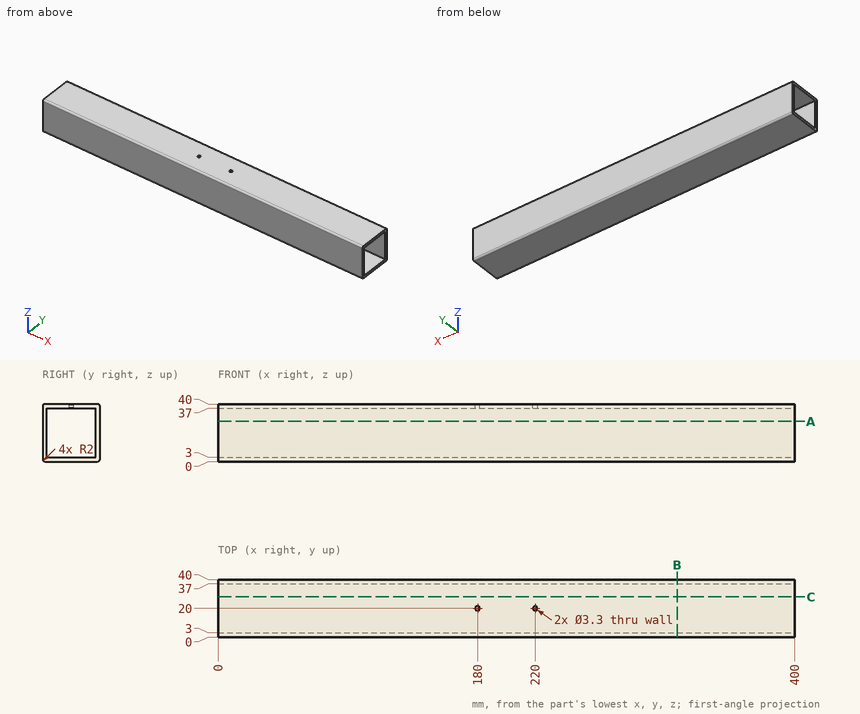
Print and shaded views of the part. All mm, measured from the part's lowest x, y and z. Give positions to 0.01 mm unless a question says otherwise; leave off trailing zeros. Loops run counter-clockwise (first coordinate to the right, second up) from the corner with the lowest first, then second, coordinate; pieces in that order, holes last. Notation, with made-up numbers: (78, 33) - (101, 33) arc R10 cw to (101, 49) - close; hole circle Ø4 at (76.25, -27.5). An arc over 180 degrees is marked (long way). One line per item, written item: value. Start each with the question number.
1. Slice it at B-B (x = 318.5). List the corners of the cut face in (y, z), plus the area to 3 significant figures.
2. Pin check, flat tips, straight feed: pin 1 (6 mm diameter, centred on y = 16, z = 7.5, fed in from +X); pin 2 (2.5 mm diameter, centred on x = 220, y = 20, fed in from +Z). Stop position of each tip, or through.
3. Slice it at A-A (z = 28). List the corners of the cut face in (x, y).
4. Probe L1, parallel to X at y = 20, z = 38; L2, parallel to Y at x = 135.5, z = 7. List the from-to ranges inside material, lowest first. Write a range as from..to.
Solution:
1. outline: (0, 2) arc R2 ccw to (2, 0) - (38, 0) arc R2 ccw to (40, 2) - (40, 38) arc R2 ccw to (38, 40) - (2, 40) arc R2 ccw to (0, 38) - close; hole (3, 3) - (37, 3) - (37, 37) - (3, 37) - close
1. area: 441 mm^2
2. pin 1: passes through
2. pin 2: stops at z = 3
3. outline: (0, 0) - (400, 0) - (400, 3) - (0, 3) - close; (0, 37) - (400, 37) - (400, 40) - (0, 40) - close
4. L1: x = 0..178.35, 181.65..218.35, 221.65..400
4. L2: y = 0..3, 37..40
